```python
from build123d import *

# Parameters (mm, degrees)
F0_R     = 30
F1_DEPTH = 5
F3_R     = 5
F4_DEPTH = 2
F5_W     = 14.7
F5_H     = 16.5
F6_DEPTH = 1.7


# Not quite as in the source:
# - a fillet or chamfer that OpenCascade refuses, or shapes differently, is made with other operations: its cross-section is extruded or revolved along the edge and cut away or added


with BuildPart() as f1:
    # F0 (on Top) → F1 (new body)
    with BuildSketch(Plane.XY):
        Circle(F0_R)
    extrude(amount=F1_DEPTH)

    # F2: fillet of radius 28.7648476108 on 1 edges, made by hand

    # F2_s1 → F2_t2 (revolve, cut)
    with BuildSketch(Plane.XZ):
        with BuildLine():
            ThreePointArc((30, 0), (22.2736681867, 3.7215915737), (13.7935668295, 5))
            Line((13.7935668295, 5), (30, 5))
            Line((30, 5), (30, 0))
        make_face()
    revolve(axis=Axis((0, 0, 5), (0, 0, 1)), mode=Mode.SUBTRACT)

    # F3 (on face) → F4 (join)
    with BuildSketch(Plane.XY.offset(5)):
        Circle(F3_R)
    extrude(amount=F4_DEPTH)

    # F5 (on face) → F6 (cut)
    with BuildSketch(Plane(origin=(0, 0, 0), x_dir=(1, 0, 0), z_dir=(0, 0, -1))):
        Rectangle(F5_W, F5_H)
    extrude(amount=-F6_DEPTH, mode=Mode.SUBTRACT)

    # F7: fillet of radius 5 on 1 edges, made by hand

    # F7_s1 → F7_t2 (revolve, cut)
    with BuildSketch(Plane.XZ):
        with BuildLine():
            ThreePointArc((5, 5), (3.2360679775, 6.472135955), (1, 7))
            Line((1, 7), (5, 7))
            Line((5, 7), (5, 5))
        make_face()
    revolve(axis=Axis((0, 0, 7), (0, 0, 1)), mode=Mode.SUBTRACT)


solid = f1.part
```
Build history of the part. All positions in model axes, mm. A direction names the side the tool comes from. Round coordinates to 2 decimals unless told otherwise and drop trailing zeros.
1) 3-axis set-ups, long thin cutter, end or side, ignore diameter. For faces 1 (the flat face through (0, 0, 7)), 2 (the flat face through (0, 0, 1.7)), 3 (the flat face through (6, 0, 5)): which of +Z, -Z, +X, -X, +Y, -Y reach the whole face in a straight line?
2) Pin check, flat tips, straight feed: pin 1 (3 mm diameter, centred on x = 19.5, z = 1.5, fed in from +Y); pin 2 (1.5 mm diameter, centred on y = 10, z = 1, fed in from +X); pin 3 (1.4 mm diameter, centred on x = -3.5, z = 1, fed in from -Y). Stop position of each tip, or through.
3) Drill centre lines: probe 1 along Z at (x, y) = (-6, 7); probe 2 along Z at (x, y) = (-10, 8.5); probe 3 along X at (y, z) = (7.5, 0.75). Where is each one in solid material? Low to high.
4) Mould opens along X. For faces 4 (the flat face through (7.35, 0, 1)), 5 (the flat face through (13, 0, 0)) say: +X half, -X half, draft (parallel to the pull), parting line (faces both ways), or undercut.
Ans:
1. face 1: +Z, +X, -X, +Y, -Y
1. face 2: -Z
1. face 3: +Z
2. pin 1: stops at y = 23.06
2. pin 2: stops at x = 27.92
2. pin 3: stops at y = -29.35
3. probe 1: z = 1.7 to 5
3. probe 2: z = 0 to 5
3. probe 3: x = -27.85 to -7.35, 7.35 to 27.85
4. face 4: undercut
4. face 5: draft
